from build123d import *

# Parameters (mm, degrees)
BASE_FLANGE1_DEPTH             = 85.725
CUT_EXTRUDE1_REACH             = 122.047
SKETCH3_R                      = 2.1082
CUT_EXTRUDE2_REACH             = 122.047
SKETCH4_R                      = 2.1082
F_4_40_TAPPED_HOLE1_AT_2_COUNT = 2
F_4_40_TAPPED_HOLE1_AT_2_PITCH = 101.6
F_4_40_TAPPED_HOLE1_AT_3_COUNT = 2
F_4_40_TAPPED_HOLE1_AT_3_PITCH = 38.1
F_4_40_TAPPED_HOLE1_AT_4_COUNT = 2
F_4_40_TAPPED_HOLE1_AT_4_PITCH = 63.5
F_4_40_TAPPED_HOLE1_AT_5_COUNT = 2
F_4_40_TAPPED_HOLE1_AT_5_PITCH = 108.508847566
F_4_40_TAPPED_HOLE1_AT_6_COUNT = 2
F_4_40_TAPPED_HOLE1_AT_6_PITCH = 50.8
FILLET1_R                      = 3.175


# Sheet-metal steps are written as plain solids
with BuildPart() as part:
    # Sketch1 → Base-Flange1 (new, symmetric)
    with BuildSketch(Plane(origin=(0, 0, 0), x_dir=(1, 0, 0), z_dir=(0, 1, 0))):
        with BuildLine():
            Line((73.8378, -2.032), (60.2996, -2.032))
            ThreePointArc((60.2996, -2.032), (59.760784633, -2.255184633), (59.5376, -2.794))
            Line((59.5376, -2.794), (59.5376, -37.338))
            ThreePointArc((59.5376, -37.338), (58.719256347, -39.313656347), (56.7436, -40.132))
            Line((56.7436, -40.132), (-56.7436, -40.132))
            ThreePointArc((-56.7436, -40.132), (-58.719256347, -39.313656347), (-59.5376, -37.338))
            Line((-59.5376, -37.338), (-59.5376, -2.794))
            ThreePointArc((-59.5376, -2.794), (-59.760784633, -2.255184633), (-60.2996, -2.032))
            Line((-60.2996, -2.032), (-73.8378, -2.032))
            Line((-73.8378, -2.032), (-73.8378, 0))
            Line((-73.8378, 0), (-60.2996, 0))
            ThreePointArc((-60.2996, 0), (-58.323943653, -0.818343653), (-57.5056, -2.794))
            Line((-57.5056, -2.794), (-57.5056, -37.338))
            ThreePointArc((-57.5056, -37.338), (-57.282415367, -37.876815367), (-56.7436, -38.1))
            Line((-56.7436, -38.1), (56.7436, -38.1))
            ThreePointArc((56.7436, -38.1), (57.282415367, -37.876815367), (57.5056, -37.338))
            Line((57.5056, -37.338), (57.5056, -2.794))
            ThreePointArc((57.5056, -2.794), (58.323943653, -0.818343653), (60.2996, 0))
            Line((60.2996, 0), (73.8378, 0))
            Line((73.8378, 0), (73.8378, -2.032))
        make_face()
    extrude(amount=BASE_FLANGE1_DEPTH, both=True)

    # Sketch3 → Cut-Extrude1 (cut, up to next)
    with BuildSketch(Plane.XY.offset(40.132), mode=Mode.PRIVATE) as cut_extrude1_sk1:
        with Locations((52.4002, 77.8002)):
            Circle(SKETCH3_R)
    cut_extrude1_tool1 = extrude(cut_extrude1_sk1.sketch, amount=-CUT_EXTRUDE1_REACH, mode=Mode.PRIVATE) & part.part
    # Sketch3 → Cut-Extrude1 (cut, up to next)
    with BuildSketch(Plane.XY.offset(40.132), mode=Mode.PRIVATE) as cut_extrude1_sk2:
        with Locations((52.4002, -77.7748)):
            Circle(SKETCH3_R)
    cut_extrude1_tool2 = extrude(cut_extrude1_sk2.sketch, amount=-CUT_EXTRUDE1_REACH, mode=Mode.PRIVATE) & part.part
    # Sketch3 → Cut-Extrude1 (cut, up to next)
    with BuildSketch(Plane.XY.offset(40.132), mode=Mode.PRIVATE) as cut_extrude1_sk3:
        with Locations((-52.3748, 77.8002)):
            Circle(SKETCH3_R)
    cut_extrude1_tool3 = extrude(cut_extrude1_sk3.sketch, amount=-CUT_EXTRUDE1_REACH, mode=Mode.PRIVATE) & part.part
    # Sketch3 → Cut-Extrude1 (cut, up to next)
    with BuildSketch(Plane.XY.offset(40.132), mode=Mode.PRIVATE) as cut_extrude1_sk4:
        with Locations((-52.3748, -77.7748)):
            Circle(SKETCH3_R)
    cut_extrude1_tool4 = extrude(cut_extrude1_sk4.sketch, amount=-CUT_EXTRUDE1_REACH, mode=Mode.PRIVATE) & part.part
    # Sketch3 → Cut-Extrude1 (cut, up to next)
    with BuildSketch(Plane.XY.offset(40.132), mode=Mode.PRIVATE) as cut_extrude1_sk5:
        with Locations((0, 77.8002)):
            Circle(SKETCH3_R)
    cut_extrude1_tool5 = extrude(cut_extrude1_sk5.sketch, amount=-CUT_EXTRUDE1_REACH, mode=Mode.PRIVATE) & part.part
    # Sketch3 → Cut-Extrude1 (cut, up to next)
    with BuildSketch(Plane.XY.offset(40.132), mode=Mode.PRIVATE) as cut_extrude1_sk6:
        with Locations((0, -77.7748)):
            Circle(SKETCH3_R)
    cut_extrude1_tool6 = extrude(cut_extrude1_sk6.sketch, amount=-CUT_EXTRUDE1_REACH, mode=Mode.PRIVATE) & part.part
    add(cut_extrude1_tool1.solids().sort_by_distance((52.4002, 77.8002, 40.132))[0], mode=Mode.SUBTRACT)
    add(cut_extrude1_tool2.solids().sort_by_distance((52.4002, -77.7748, 40.132))[0], mode=Mode.SUBTRACT)
    add(cut_extrude1_tool3.solids().sort_by_distance((-52.3748, 77.8002, 40.132))[0], mode=Mode.SUBTRACT)
    add(cut_extrude1_tool4.solids().sort_by_distance((-52.3748, -77.7748, 40.132))[0], mode=Mode.SUBTRACT)
    add(cut_extrude1_tool5.solids().sort_by_distance((0, 77.8002, 40.132))[0], mode=Mode.SUBTRACT)
    add(cut_extrude1_tool6.solids().sort_by_distance((0, -77.7748, 40.132))[0], mode=Mode.SUBTRACT)

    # Sketch4 → Cut-Extrude2 (cut, up to next)
    with BuildSketch(Plane.XY, mode=Mode.PRIVATE) as cut_extrude2_sk1:
        with Locations((65.1002, -77.7748)):
            Circle(SKETCH4_R)
    cut_extrude2_tool1 = extrude(cut_extrude2_sk1.sketch, amount=CUT_EXTRUDE2_REACH, mode=Mode.PRIVATE) & part.part
    # Sketch4 → Cut-Extrude2 (cut, up to next)
    with BuildSketch(Plane.XY, mode=Mode.PRIVATE) as cut_extrude2_sk2:
        with Locations((65.1002, 77.8002)):
            Circle(SKETCH4_R)
    cut_extrude2_tool2 = extrude(cut_extrude2_sk2.sketch, amount=CUT_EXTRUDE2_REACH, mode=Mode.PRIVATE) & part.part
    # Sketch4 → Cut-Extrude2 (cut, up to next)
    with BuildSketch(Plane.XY, mode=Mode.PRIVATE) as cut_extrude2_sk3:
        with Locations((-65.0748, 77.8002)):
            Circle(SKETCH4_R)
    cut_extrude2_tool3 = extrude(cut_extrude2_sk3.sketch, amount=CUT_EXTRUDE2_REACH, mode=Mode.PRIVATE) & part.part
    # Sketch4 → Cut-Extrude2 (cut, up to next)
    with BuildSketch(Plane.XY, mode=Mode.PRIVATE) as cut_extrude2_sk4:
        with Locations((-65.0748, -77.7748)):
            Circle(SKETCH4_R)
    cut_extrude2_tool4 = extrude(cut_extrude2_sk4.sketch, amount=CUT_EXTRUDE2_REACH, mode=Mode.PRIVATE) & part.part
    # Sketch4 → Cut-Extrude2 (cut, up to next)
    with BuildSketch(Plane.XY, mode=Mode.PRIVATE) as cut_extrude2_sk5:
        with Locations((65.1002, 0)):
            Circle(SKETCH4_R)
    cut_extrude2_tool5 = extrude(cut_extrude2_sk5.sketch, amount=CUT_EXTRUDE2_REACH, mode=Mode.PRIVATE) & part.part
    # Sketch4 → Cut-Extrude2 (cut, up to next)
    with BuildSketch(Plane.XY, mode=Mode.PRIVATE) as cut_extrude2_sk6:
        with Locations((-65.0748, 0)):
            Circle(SKETCH4_R)
    cut_extrude2_tool6 = extrude(cut_extrude2_sk6.sketch, amount=CUT_EXTRUDE2_REACH, mode=Mode.PRIVATE) & part.part
    add(cut_extrude2_tool1.solids().sort_by_distance((65.1002, -77.7748, 0))[0], mode=Mode.SUBTRACT)
    add(cut_extrude2_tool2.solids().sort_by_distance((65.1002, 77.8002, 0))[0], mode=Mode.SUBTRACT)
    add(cut_extrude2_tool3.solids().sort_by_distance((-65.0748, 77.8002, 0))[0], mode=Mode.SUBTRACT)
    add(cut_extrude2_tool4.solids().sort_by_distance((-65.0748, -77.7748, 0))[0], mode=Mode.SUBTRACT)
    add(cut_extrude2_tool5.solids().sort_by_distance((65.1002, 0, 0))[0], mode=Mode.SUBTRACT)
    add(cut_extrude2_tool6.solids().sort_by_distance((-65.0748, 0, 0))[0], mode=Mode.SUBTRACT)

    # Sketch5 → #4-40 Tapped Hole1 (revolve, cut)
    with BuildSketch(Plane(origin=(52.4256, -50.8, 40.132), x_dir=(0, -1, 0), z_dir=(1, 0, 0))):
        Polygon((0, 0), (0, 2.032), (1.4986, 2.032), (1.1303, 1.6637), (1.1303, 0.3683), (1.4986, 0), align=None)
    f_4_40_tapped_hole1 = revolve(axis=Axis((52.4256, -50.8, 46.482), (0, 0, -1)), mode=Mode.SUBTRACT)

    # #4-40 Tapped Hole1 at 2: #4-40 Tapped Hole1 ×2
    with Locations(*[(0, i * F_4_40_TAPPED_HOLE1_AT_2_PITCH, 0) for i in range(1, F_4_40_TAPPED_HOLE1_AT_2_COUNT)]):
        add(f_4_40_tapped_hole1, mode=Mode.SUBTRACT)

    # #4-40 Tapped Hole1 at 3: #4-40 Tapped Hole1 ×2
    with Locations(*[(-i * F_4_40_TAPPED_HOLE1_AT_3_PITCH, 0, 0) for i in range(1, F_4_40_TAPPED_HOLE1_AT_3_COUNT)]):
        add(f_4_40_tapped_hole1, mode=Mode.SUBTRACT)

    # #4-40 Tapped Hole1 at 4: #4-40 Tapped Hole1 ×2
    with Locations(*[Vector(-0.6000000000000001, 0.8, 0) * (i * F_4_40_TAPPED_HOLE1_AT_4_PITCH) for i in range(1, F_4_40_TAPPED_HOLE1_AT_4_COUNT)]):
        add(f_4_40_tapped_hole1, mode=Mode.SUBTRACT)

    # #4-40 Tapped Hole1 at 5: #4-40 Tapped Hole1 ×2
    with Locations(*[Vector(-0.35112344158839176, 0.9363291775690445, 0) * (i * F_4_40_TAPPED_HOLE1_AT_5_PITCH) for i in range(1, F_4_40_TAPPED_HOLE1_AT_5_COUNT)]):
        add(f_4_40_tapped_hole1, mode=Mode.SUBTRACT)

    # #4-40 Tapped Hole1 at 6: #4-40 Tapped Hole1 ×2
    with Locations(*[(0, i * F_4_40_TAPPED_HOLE1_AT_6_PITCH, 0) for i in range(1, F_4_40_TAPPED_HOLE1_AT_6_COUNT)]):
        add(f_4_40_tapped_hole1, mode=Mode.SUBTRACT)

    # Fillet1
    fillet1_edges = [part.edges().sort_by_distance(p)[0] for p in [
        (73.8378, -85.725, 1.016),
        (-73.8378, -85.725, 1.016),
        (73.8378, 85.725, 1.016),
        (-73.8378, 85.725, 1.016),
    ]]
    fillet(fillet1_edges, radius=FILLET1_R)


solid = part.part
Can you work these out from the model? Positions are in its coordinate system, mm. A direction names the side the tool comes from. Give positions to 0.01 mm unless a question says otherwise; leave off trailing zeros. Order: outer loops, then holes, each group sorted by start corner. A loop starts at its lowest first (then second) coordinate and runs counter-clockwise, first axis right, second up. Notation, with made-up numbers: M 59,-6 L 76,-6 A20 cw 76,25 Z; hole C 38,18.5 d3. An arc over 180 degrees is marked long. Use one line per item in the form item = value. Start each with the question number.
Item 1: If we section it at B-B (x = 0): Write out the boundary of the cut face in (y, z) (3 decimals), then the cut area to 3 significant figures.
Item 2: We'd pull the mould along X, two halves only. Please class faces 1 (the flat face through (68, 1, 0)), 2 (the flat face through (-59.538, 1, 20)), 3 (the flat face through (-1, 1, 38.1)): +X half, -X half, draft (parallel to the pull), parting line (faces both ways), or undercut.
Item 3: If I drill on line 1 along Y through (x, z) = (0, 38.85) (3 decimals); line 2 along X through (y, z) = (32, 35.5); line 3 along X through (y, z) = (50.8, 39.5), over which ranges is the centre line in solid material (lowest first)?
Item 4: If we section it at C-C (y = -9): Write out the boundary of the cut face in (x, z).
Item 5: Will these pins go through, and if not, where does the flat tip stop? pin 1 Ø4 at (y, z) = (-57, 25) entering from -X; pin 2 Ø15 at (x, y) = (-69.5, -9) entering from +Z; pin 3 Ø10 at (x, y) = (-22, 3) entering from -Z.
Item 6: For faces 4 (the flat face through (67.2, 1.2, 2.032)), 5 (the flat face through (-67, 1.2, 2.032)), 6 (the flat face through (1, 1, 40.132)), which set-ups out of +Z, -Z, +X, -X, +Y, -Y let a thin tool reach every point of the face, with its end or its side?
Item 7: If we section it at A-A (z = 24): Write out the boundary of the cut face in (x, y) (3 decimals).
Outcome:
q1.outline = M -85.725,38.1 L -79.883,38.1 L -79.883,40.132 L -85.725,40.132 Z; M -75.667,38.1 L 75.692,38.1 L 75.692,40.132 L -75.667,40.132 Z; M 79.908,38.1 L 85.725,38.1 L 85.725,40.132 L 79.908,40.132 Z
q1.area = 331 mm2
q2.face_1 = draft
q2.face_2 = -X half
q2.face_3 = undercut
q3.line_1 = -85.725 to -79.883, -75.667 to 75.692, 79.908 to 85.725
q3.line_2 = -59.54 to -57.51, 57.51 to 59.54
q3.line_3 = -58.51 to 13.2, 15.46 to 51.3, 53.56 to 58.51
q4.outline = M -73.84,0 L -60.3,0 A2.79 ccw -57.51,2.79 L -57.51,37.34 A0.76 cw -56.74,38.1 L 56.74,38.1 A0.76 cw 57.51,37.34 L 57.51,2.79 A2.79 ccw 60.3,0 L 73.84,0 L 73.84,2.03 L 60.3,2.03 A0.76 cw 59.54,2.79 L 59.54,37.34 A2.79 ccw 56.74,40.13 L -56.74,40.13 A2.79 ccw -59.54,37.34 L -59.54,2.79 A0.76 cw -60.3,2.03 L -73.84,2.03 Z
q5.pin_1 = -59.54
q5.pin_2 = 2.03
q5.pin_3 = 38.1
q6.face_4 = +Z, +X, +Y, -Y
q6.face_5 = +Z, -X, +Y, -Y
q6.face_6 = +Z, +X, -X, +Y, -Y
q7.outline = M -59.538,-85.725 L -57.506,-85.725 L -57.506,85.725 L -59.538,85.725 Z; M 57.506,-85.725 L 59.538,-85.725 L 59.538,85.725 L 57.506,85.725 Z
